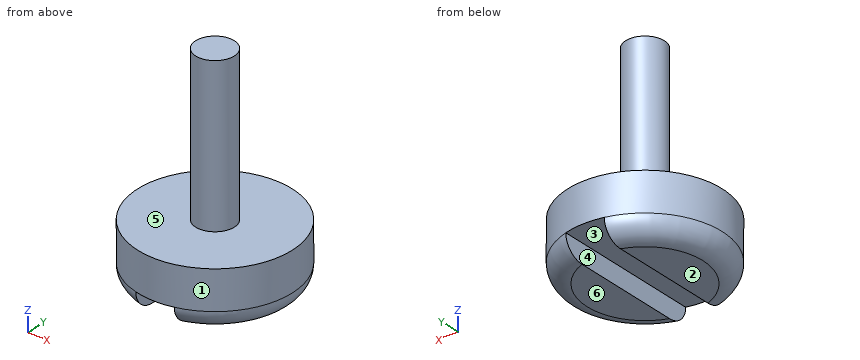
from build123d import *

# Parameters (mm, degrees)
F0_R     = 4
F1_DEPTH = 3
F2_R     = 1
F3_DEPTH = 8
F4_W     = 2
F4_H     = 10.9652710235
F5_DEPTH = 1
F6_R     = 1


with BuildPart() as f1:
    # F0 (on Top) → F1 (new body)
    with BuildSketch(Plane.XY):
        Circle(F0_R)
    extrude(amount=F1_DEPTH)

    # F2 (on face) → F3 (join)
    with BuildSketch(Plane.XY.offset(3)):
        Circle(F2_R)
    extrude(amount=F3_DEPTH)

    # F4 (on face) → F5 (cut)
    with BuildSketch(Plane(origin=(0, 0, 0), x_dir=(1, 0, 0), z_dir=(0, 0, -1))):
        Rectangle(F4_W, F4_H)
    extrude(amount=-F5_DEPTH, mode=Mode.SUBTRACT)

    # F6
    f6_edges = [f1.edges().sort_by_distance(p)[0] for p in [
        (-4, 0, 0),
        (3.162278, 2.44949, 0),
        (3.162278, -2.44949, 0),
    ]]
    fillet(f6_edges, radius=F6_R)


solid = f1.part
Geometry check sheet. Reference: the model listing, model coordinates, mm. Face numbers are marked on the shaded views. A direction names the side the tool comes from. Round coordinates to 2 decimals unless told otherwise and drop trailing zeros. Order: outer loops, then holes, each group sorted by start corner. A loop starts at its lowest first (then second) coordinate and runs counter-clockwise, first axis right, second up. Notation, with made-up numbers: M 4.5,14 L 10.5,14 A28 cw 10.5,32 Z; hole C 60.25,-10 d2. An arc over 180 degrees is marked long. Answer in a Markdown table with one row per item. Add a question column.
Item 1: Sectioned sample at A-A, the plane x = 0. Enter the section's corners in (y, z).
Item 2: Depth check by flat-ended pin: pin 1 Ø1 at (y, z) = (-2.5, 2) entering from +X; pin 2 Ø3 at (x, z) = (2, 8.5) entering from -Y; pin 3 Ø0.5 at (y, z) = (-0.5, 0.5) entering from -X. Enter the tip coordinate at first touch or a pass-through.
Item 3: Draft check along X on the marked faces 1, 2 and 3. Enter one of: released by +X, released by -X, zero draft, split by the parting line, or undercut.
Item 4: Material ranges on L1, parallel to Y at x = 1, z = 2; L2, parallel to Z at x = 2.5, y = -0.25; L3, parallel to Z at x = -0.75, y = 0, recorded low to high. Write a range as [from, to].
Item 5: Sectioned sample at B-B, the plane y = 0. Enter the section's corners in (x, z).
Item 6: Sectioned sample at C-C, the plane z = 4. Enter the section's corners in (x, y), plus the area to 3 significant figures.
Item 7: Set-up check for the marked faces 4, 5 and 6: record each of +Z, -Z, +X, -X, +Y, -Y from which the full face is reachable in a straight line by a thin tool's end or side.
Filled in:
| question | item | result |
|---|---|---|
| 1 | outline | M -4,1 L 4,1 L 4,3 L 1,3 L 1,11 L -1,11 L -1,3 L -4,3 Z |
| 2 | pin 1 | stops at x = 3.46 |
| 2 | pin 2 | stops at y = -0.87 |
| 2 | pin 3 | stops at x = -3.94 |
| 3 | face 1 | split by the parting line |
| 3 | face 2 | zero draft |
| 3 | face 3 | undercut |
| 4 | L1 | y = [-3.87, 3.87] |
| 4 | L2 | z = [0, 3] |
| 4 | L3 | z = [1, 11] |
| 5 | outline | M -4,1 A1 ccw -3,0 L -1,0 L -1,1 L 1,1 L 1,0 L 3,0 A1 ccw 4,1 L 4,3 L 1,3 L 1,11 L -1,11 L -1,3 L -4,3 Z |
| 6 | outline | C 0,0 d2 |
| 6 | area | 3.14 mm² |
| 7 | face 4 | -Z, +Y, -Y |
| 7 | face 5 | +Z |
| 7 | face 6 | -Z, +X, -X, +Y, -Y |
